Autodesk Inventor part; units mm, degrees
ref_plane "YZ Plane" through (0, 0, 0) normal (1, 0, 0) x (0, 1, 0)
ref_plane "XZ Plane" through (0, 0, 0) normal (0, 1, 0) x (-1, 0, 0)
ref_plane "XY Plane" through (0, 0, 0) normal (0, 0, 1) x (1, 0, 0)
sketch "Sketch6" plane through (0, 0, 0) normal (0, 1, 0) x (-1, 0, 0)
  line L0 (407.1, -490) -> (-407.1, -490)
  line L1 (-407.1, -490) -> (-407.1, 490)
  line L2 (-407.1, 490) -> (407.1, 490)
  line L3 (407.1, 490) -> (407.1, -490)
  line L4 (407.1, -490) -> (-407.1, 490) construction
  line L5 (-407.1, -490) -> (407.1, 490) construction
  point P0 (0, 0)
  dimension "d52" = 814.2
  dimension "d53" = 980
extrude "Plate2" add sketch "Sketch6" along normal blind 0.5
sketch "Sketch11" plane through (406.6, 0, -490) normal (1, 0, 0) x (0, 1, 0)
  line L0 (0, 980) -> (0, 0)
  line L1 (0, 0) -> (10, 0)
  line L2 (10, 0) -> (10, 980)
  line L3 (10, 980) -> (0, 980)
edge flange "Flange2" height 10 angle 90 thickness 0.5 bend radius 0.5 thickness toward (1, 0, 0) relief tear relief width 0.5 relief depth 0.25 edges at (407.1, 0.5, 0) wall of the first edge with corners at (406.6, 0, 490) (406.6, 0, -490) (406.6, 10, -490) (406.6, 10, 490)
bend "Bend3"
corner "Corner3"
sketch "Sketch12" plane through (407.1, 9.5, -490) normal (0, 1, 0) x (-1, 0, 0)
  line L0 (0, 980) -> (0, 0)
  line L1 (0, 0) -> (10, 0)
  line L2 (10, 0) -> (10, 980)
  line L3 (10, 980) -> (0, 980)
edge flange "Flange3" height 10 angle 90 thickness 0.5 bend radius 0.5 thickness toward (0, 1, 0) relief tear relief width 0.5 relief depth 0.25 edges at (406.6, 10, 0) wall of the first edge with corners at (407.1, 9.5, 490) (407.1, 9.5, -490) (397.1, 9.5, -490) (397.1, 9.5, 490)
bend "Bend4"
corner "Corner4"
sketch "Sketch13" plane through (-406.6, 0, 490) normal (-1, 0, 0) x (0, -1, 0)
  line L0 (0, -980) -> (0, 0)
  line L1 (0, 0) -> (-10, 0)
  line L2 (-10, 0) -> (-10, -980)
  line L3 (-10, -980) -> (0, -980)
edge flange "Flange4" height 10 angle 90 thickness 0.5 bend radius 0.5 thickness toward (-1, 0, 0) relief tear relief width 0.5 relief depth 0.25 edges at (-407.1, 0.5, 0) wall of the first edge with corners at (-406.6, 0, -490) (-406.6, 0, 490) (-406.6, 10, 490) (-406.6, 10, -490)
bend "Bend5"
corner "Corner5"
sketch "Sketch14" plane through (-407.1, 9.5, 490) normal (0, 1, 0) x (-1, 0, 0)
  line L0 (0, -980) -> (0, 0)
  line L1 (0, 0) -> (-10, 0)
  line L2 (-10, 0) -> (-10, -980)
  line L3 (-10, -980) -> (0, -980)
edge flange "Flange5" height 10 angle 90 thickness 0.5 bend radius 0.5 thickness toward (0, 1, 0) relief tear relief width 0.5 relief depth 0.25 edges at (-406.6, 10, 0) wall of the first edge with corners at (-407.1, 9.5, -490) (-407.1, 9.5, 490) (-397.1, 9.5, 490) (-397.1, 9.5, -490)
bend "Bend6"
corner "Corner6"
equation "\"d52\" = ЖАБРЫ_базовая_ширина - ЖАБРЫ_шаг_листов"
equation "\"d53\" = ЖАБРЫ_базовая_длина_кор_лист"
equation "\"d54\" = Thickness"
equation "\"d84\" = BendReliefWidth"
equation "\"d85\" = BendReliefDepth"
equation "\"d86\" = MinimumRemnant"
equation "\"d87\" = TransitionRadius"
equation "\"d90\" = BendRadius"
equation "\"d91\" = CornerReliefSize"
equation "\"d92\" = GapSize"
equation "\"d93\" = JacobiRadiusSize"
equation "\"d94\" = BendReliefWidth"
equation "\"d95\" = BendReliefDepth"
equation "\"d96\" = MinimumRemnant"
equation "\"d97\" = TransitionRadius"
equation "\"d100\" = BendRadius"
equation "\"d101\" = CornerReliefSize"
equation "\"d102\" = GapSize"
equation "\"d103\" = JacobiRadiusSize"
equation "\"d104\" = BendReliefWidth"
equation "\"d105\" = BendReliefDepth"
equation "\"d106\" = MinimumRemnant"
equation "\"d107\" = TransitionRadius"
equation "\"d110\" = BendRadius"
equation "\"d111\" = CornerReliefSize"
equation "\"d112\" = GapSize"
equation "\"d113\" = JacobiRadiusSize"
equation "\"d114\" = BendReliefWidth"
equation "\"d115\" = BendReliefDepth"
equation "\"d116\" = MinimumRemnant"
equation "\"d117\" = TransitionRadius"
equation "\"d120\" = BendRadius"
equation "\"d121\" = CornerReliefSize"
equation "\"d122\" = GapSize"
equation "\"d123\" = JacobiRadiusSize"
equation "\"BendRadius\" = Thickness"
equation "\"BendReliefWidth\" = Thickness"
equation "\"BendReliefDepth\" = 0.5 * Thickness"
equation "\"CornerReliefSize\" = 4 * Thickness"
equation "\"MinimumRemnant\" = 2 * Thickness"
equation "\"TransitionRadius\" = BendRadius"
equation "\"JacobiRadiusSize\" = BendRadius"
equation "\"GapSize\" = Thickness"
properties part number "MSC 803 sheet gills" material "Stainless Steel"
Can you work these out from the model? Positions are in its coordinate system, mm. Give positions to 0.01 mm unless a question says otherwise; leave off trailing zeros. Order: outer loops, then holes, each group sorted by start corner. A loop starts at its lowest first (then second) coordinate and runs counter-clockwise, first axis right, second up. Notation, with made-up numbers: (-26.5, 20.5) - (17.5, 20.5) arc R9 ccw to (17.5, 27.5) - close; hole circle Ø5 at (-1.75, -15.75). An arc over 180 degrees is marked (long way). Use a Markdown table: item, result. Add a question column.
Q1. If we section it at B-B on z = 262.5: Write out the boundary of the cut face in (x, y), plus the area to 3 significant figures.
Q2. If we mould it in two halves opening along X, with no side actions, what happens to faces 1 (the flat face through (6, 0.5, 7)), 2 (the flat face through (6, 0, 7))? For each: released by +X, released by -X, zero draft, split by the parting line, or undercut.
Q3. Please list where these lines run through material, in increasing order: line 1 along X through (y, z) = (2.5, -440); line 2 along X through (y, z) = (9.25, 76.5); line 3 along Y through (x, z) = (367.5, 3).
Q4. If we section it at A-A on y = 6.25: Write out the boundary of the cut face in (x, z).
Q5. If we section it at C-C on x = -138: Write out the boundary of the cut face in (y, z).
Q6. I'm going to push flat-ended pins straight in: pin 1 (10 mm diameter, centred on x = 160.5, z = -378, fed in from -Y); pin 2 (3 mm diameter, centred on x = 79, z = 42, fed in from +Y); pin 3 (0.6 mm diameter, centred on y = 9.5, z = 22, fed in from +X). Where does each tip first touch, or does it pass through?
Answers follow:
| question | item | result |
|---|---|---|
| 1 | outline | (-407.1, 1) arc R1 ccw to (-406.1, 0) - (406.1, 0) arc R1 ccw to (407.1, 1) - (407.1, 9) arc R1 ccw to (406.1, 10) - (397.1, 10) - (397.1, 9.5) - (406.1, 9.5) arc R0.5 cw to (406.6, 9) - (406.6, 1) arc R0.5 cw to (406.1, 0.5) - (-406.1, 0.5) arc R0.5 cw to (-406.6, 1) - (-406.6, 9) arc R0.5 cw to (-406.1, 9.5) - (-397.1, 9.5) - (-397.1, 10) - (-406.1, 10) arc R1 ccw to (-407.1, 9) - close |
| 1 | area | 425 mm^2 |
| 2 | face 1 | undercut |
| 2 | face 2 | zero draft |
| 3 | line 1 | x = -407.1 to -406.6, 406.6 to 407.1 |
| 3 | line 2 | x = -407.07 to -406.53, 406.53 to 407.07 |
| 3 | line 3 | y = 0 to 0.5 |
| 4 | outline | (-407.1, -490) - (-406.6, -490) - (-406.6, 490) - (-407.1, 490) - close; (406.6, -490) - (407.1, -490) - (407.1, 490) - (406.6, 490) - close |
| 5 | outline | (0, -490) - (0.5, -490) - (0.5, 490) - (0, 490) - close |
| 6 | pin 1 | stops at y = 0 |
| 6 | pin 2 | stops at y = 0.5 |
| 6 | pin 3 | stops at x = 407.08 |
